Design review of the part built by this model. Coordinates are the model's own, in mm. Face numbers are marked on the shaded views. A direction names the side the tool comes from. Give positions to 0.01 mm unless a question says otherwise; leave off trailing zeros. Loops run counter-clockwise (first coordinate to the right, second up) from the corner with the lowest first, then second, coordinate; pieces in that order, holes last.
from build123d import *

# Parameters (mm, degrees)
SKETCH_1_R          = 5
SKETCH_1_R_2        = 2.5
EXTRUDE_1_DEPTH     = 7.5
SKETCH_2_R          = 4.5
SKETCH_2_R_2        = 3
CUT_EXTRUDE_1_DEPTH = 0.15


with BuildPart() as part:
    # Эскиз1 → Бобышка-Вытянуть1 (new body)
    with BuildSketch(Plane(origin=(0, 0, 0), x_dir=(1, 0, 0), z_dir=(0, 1, 0))):
        with Locations(Location((0, 0, 0), (0, 0, 270))):
            Circle(SKETCH_1_R)
        with Locations(Location((0, 0, 0), (0, 0, 270))):
            Circle(SKETCH_1_R_2, mode=Mode.SUBTRACT)
    extrude(amount=EXTRUDE_1_DEPTH)

    # Эскиз2 → Вырез-Вытянуть1 (cut)
    with BuildSketch(Plane(origin=(0, 7.5, 0), x_dir=(1, 0, 0), z_dir=(0, 1, 0))):
        with Locations(Location((0, 0, 0), (0, 0, 270))):
            Circle(SKETCH_2_R)
        with Locations(Location((0, 0, 0), (0, 0, 270))):
            Circle(SKETCH_2_R_2, mode=Mode.SUBTRACT)
    extrude(amount=-CUT_EXTRUDE_1_DEPTH, mode=Mode.SUBTRACT)

    # Зеркальное отражение1: part across plane


with BuildPart() as part_1:
    add(part.part)
    add(part.part.mirror(Plane.ZX))


solid = part_1.part
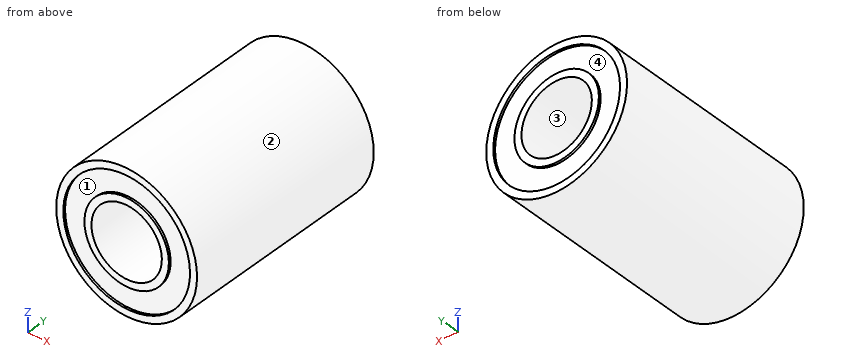
Q1. Draft analysis for pull direction X (two halves, no side actions). For the marked faces 1 and 2, state which applies: pulls with the +X half, pulls with the -X half, needs draft (parallel to the pull), parting line crosses it, or undercut.
Results:
face 1: undercut
face 2: parting line crosses it
Q2. Take a section at A-A (x = 0). Give the boundary of the cut face in (y, z), plus the area to 3 significant figures.
Results:
outline: (-7.5, -5) - (7.5, -5) - (7.5, -4.5) - (7.35, -4.5) - (7.35, -3) - (7.5, -3) - (7.5, -2.5) - (-7.5, -2.5) - (-7.5, -3) - (-7.35, -3) - (-7.35, -4.5) - (-7.5, -4.5) - close; (-7.5, 2.5) - (7.5, 2.5) - (7.5, 3) - (7.35, 3) - (7.35, 4.5) - (7.5, 4.5) - (7.5, 5) - (-7.5, 5) - (-7.5, 4.5) - (-7.35, 4.5) - (-7.35, 3) - (-7.5, 3) - close
area: 74.1 mm2
Q3. Tool access review of the marked faces 3 and 4: name each direction out of +Z, -Z, +X, -X, +Y, -Y from which nothing blocks a thin tool from reaching the whole face with its end or side.
Results:
face 3: +Y, -Y
face 4: +Y
Q4. Take a section at C-C (y = -3.75). Give the boundary of the cut face in (x, z).
Results:
outline: circle Ø10 at (0, 0); hole circle Ø5 at (0, 0)
Q5. Take a section at B-B (z = 0). Give the boundary of the cut face in (x, y), plus the area to 3 significant figures.
Results:
outline: (-5, -7.5) - (-4.5, -7.5) - (-4.5, -7.35) - (-3, -7.35) - (-3, -7.5) - (-2.5, -7.5) - (-2.5, 7.5) - (-3, 7.5) - (-3, 7.35) - (-4.5, 7.35) - (-4.5, 7.5) - (-5, 7.5) - close; (2.5, -7.5) - (3, -7.5) - (3, -7.35) - (4.5, -7.35) - (4.5, -7.5) - (5, -7.5) - (5, 7.5) - (4.5, 7.5) - (4.5, 7.35) - (3, 7.35) - (3, 7.5) - (2.5, 7.5) - close
area: 74.1 mm2
Q6. Take a section at D-D (x = 4.25). Give the boundary of the cut face in (y, z).
Results:
outline: (-7.5, -2.63) - (7.5, -2.63) - (7.5, -1.48) - (7.35, -1.48) - (7.35, 1.48) - (7.5, 1.48) - (7.5, 2.63) - (-7.5, 2.63) - (-7.5, 1.48) - (-7.35, 1.48) - (-7.35, -1.48) - (-7.5, -1.48) - close
Q7. Insertion check: pin 1 (5 mm diameter, centred on x = -3, y = 2.5, fed in from -Z); pin 2 (3 mm diameter, centred on y = -2.5, z = 2.5, fed in from +X); pin 3 (4 mm diameter, centred on y = 6, z = 2.5, fed in from +X). Each pin has a flat end and moves straight along its axis. Give the tip position at first contact, or say it passes through.
Results:
pin 1: stops at z = -4.97
pin 2: stops at x = 4.9
pin 3: stops at x = 4.97
Q8. Wall thickness on line 1 (X direction, y = -7.4, z = 0); line 2 (Y direction, x = 1, z = 4); line 3 (Z direction, x = 4, y = 6.25): over which ranges is each line inside the solid? List them lowest first.
Results:
line 1: x = -5 to -4.5, -3 to -2.5, 2.5 to 3, 4.5 to 5
line 2: y = -7.35 to 7.35
line 3: z = -3 to 3
